Part model, mm, in its own coordinate system. A direction names the side the tool comes from. Give positions to 0.01 mm unless a question says otherwise; leave off trailing zeros. Order: outer loops, then holes, each group sorted by start corner. A loop starts at its lowest first (then second) coordinate and runs counter-clockwise, first axis right, second up. Notation, with made-up numbers: M -3.75,73.5 L 35.25,73.5 A20 ccw 35.25,90.5 Z; hole C 78,35.25 d10. An arc over 180 degrees is marked long. One line per question, with ' | ' between items.
```python
from build123d import *

# Parameters (mm, degrees)
F1_DEPTH  = 76.2
F2_DEPTH  = 12.7
F3_R      = 76.19999
F6_DEPTH  = 25.401
F7_DEPTH  = 25.401
F5_W      = 38.1
F5_H      = 12.7
F5_H_2    = 25.4
F8_DEPTH  = 25.4
F9_R      = 25.4
F10_R     = 25.39999
F11_DEPTH = 12.7


# Not quite as in the source:
# - a fillet or chamfer is up to 0.001 mm smaller than in the source, because OpenCascade refuses the exact size
# - a feature names something its author has since deleted; it is built from what else it names


with BuildPart() as f1:
    # F0 (on Front) → F1 (new body, symmetric)
    with BuildSketch(Plane.XZ):
        Polygon((0, 203.2), (0, 0), (254, 0), (254, 25.4), (76.2, 25.4), (25.4, 25.4), (25.4, 76.2), (25.4, 203.2), align=None)
    extrude(amount=F1_DEPTH, both=True)

    # F0 (on Front) → F2 (join, symmetric)
    with BuildSketch(Plane.XZ):
        Polygon((76.2, 25.4), (25.4, 76.2), (25.4, 25.4), align=None)
    extrude(amount=F2_DEPTH, both=True)

    # F3 (radius 76.2 in the source; OpenCascade refuses exactly that, so slightly less here)
    f3_edges = [f1.edges().sort_by_distance(p)[0] for p in [
        (12.7, -76.2, 203.2),
        (12.7, 76.2, 203.2),
    ]]
    fillet(f3_edges, radius=F3_R)

    # F5 (on face) → F6 (cut, through all)
    with BuildSketch(Plane.XY.offset(25.4)):
        with BuildLine():
            Line((203.2, 63.5), (127, 63.5))
            ThreePointArc((127, 63.5), (114.3, 50.8), (127, 38.1))
            Line((127, 38.1), (203.2, 38.1))
            ThreePointArc((203.2, 38.1), (215.9, 50.8), (203.2, 63.5))
        make_face()
        with BuildLine():
            Line((203.2, -38.1), (127, -38.1))
            ThreePointArc((127, -38.1), (114.3, -50.8), (127, -63.5))
            Line((127, -63.5), (203.2, -63.5))
            ThreePointArc((203.2, -63.5), (215.9, -50.8), (203.2, -38.1))
        make_face()
    extrude(amount=-F6_DEPTH, mode=Mode.SUBTRACT)

    # F4 (on face) → F7 (cut, through all)
    with BuildSketch(Plane.YZ.offset(25.4)):
        with BuildLine():
            Line((0, 101.6), (0, 177.8))
            ThreePointArc((0, 177.8), (-38.1, 139.7), (0, 101.6))
        make_face()
        with BuildLine():
            ThreePointArc((0, 101.6), (26.9407683632, 112.7592316368), (38.1, 139.7))
            ThreePointArc((38.1, 139.7), (26.9407683632, 166.6407683632), (0, 177.8))
            Line((0, 177.8), (0, 101.6))
        make_face()
    extrude(amount=-F7_DEPTH, mode=Mode.SUBTRACT)

    # F5 (on face) → F8 (join)
    with BuildSketch(Plane.XY.offset(25.4)):
        with Locations((273.05, 19.05)):
            Rectangle(F5_W, F5_H)
        with Locations((273.05, -19.05)):
            Rectangle(F5_W, F5_H)
        with Locations((273.05, 0)):
            Rectangle(F5_W, F5_H_2)
    extrude(amount=-F8_DEPTH)

    # F9
    f9_edges = [f1.edges().sort_by_distance(p)[0] for p in [
        (254, 76.2, 12.7),
        (254, -76.2, 12.7),
    ]]
    fillet(f9_edges, radius=F9_R)

    # F10 (radius 25.4 in the source; OpenCascade refuses exactly that, so slightly less here)
    f10_edges = [f1.edges().sort_by_distance(p)[0] for p in [
        (254, 25.4, 12.7),
        (254, -25.4, 12.7),
    ]]
    fillet(f10_edges, radius=F10_R)

    # F5 (on face) → F11 (cut)
    with BuildSketch(Plane.XY.offset(25.4)):
        with BuildLine():
            Line((254, -12.7), (254, 12.7))
            ThreePointArc((254, 12.7), (241.3, 0), (254, -12.7))
        make_face()
        with Locations((273.05, 0)):
            Rectangle(F5_W, F5_H_2)
    extrude(amount=-F11_DEPTH, mode=Mode.SUBTRACT)


solid = f1.part
```
1. Mould opens along Y. For faces 6 (the cylindrical face through (114.303, 51.079, 12.878)), 7 (the flat face through (51.2, -0.2, 50.4)), 8 (the cylindrical face through (246.36, 68.96, 12.88)) say: released by +Y, released by -Y, zero draft, split by the parting line, or undercut.
Worked out:
face 6: undercut | face 7: zero draft | face 8: released by +Y
2. Drop flat-ended pins along their axis: pin 1 (3 mm diameter, centred on x = 87, y = -22, fed in from +Z); pin 2 (14 mm diameter, centred on x = 286.5, z = 15.5, fed in from -Y); pin 3 (6.5 mm diameter, centred on x = 271, z = 20, fed in from +Y). Give the stop position or say it passes through.
Worked out:
pin 1: stops at z = 25.4 | pin 2: stops at y = -25.4 | pin 3: stops at y = 28.23
3. Tool access for faces 1 (the flat face through (39, 12.7, 40)), 2 (the flat face through (161, -1, 25.4)), 3 (the flat face through (71, 76.2, 21)), 4 (the flat face through (166, 63.5, 13)), 5 (the flat face through (286, -25.4, 13)): list every direction of +Z, -Z, +X, -X, +Y, -Y with a clear straight run to the whole face (end or side of a thin tool).
Worked out:
face 1: +Z, +X, +Y | face 2: +Z, +X | face 3: +Z, -Z, +X, -X, +Y | face 4: +Z, -Z | face 5: +Z, -Z, +X, -Y
4. Slice it at A-A on x = 184. Give the cut face in (y, z), then the cut area to 3 significant figures.
Worked out:
outline: M -76.2,0 L -63.5,0 L -63.5,25.4 L -76.2,25.4 Z; M -38.1,0 L 38.1,0 L 38.1,25.4 L -38.1,25.4 Z; M 63.5,0 L 76.2,0 L 76.2,25.4 L 63.5,25.4 Z | area: 2,580 mm2
5. Slice it at B-B on z = 144. Give the cut face in (x, y).
Worked out:
outline: M 0,-74.28 L 25.4,-74.28 L 25.4,-37.86 L 0,-37.86 Z; M 0,37.86 L 25.4,37.86 L 25.4,74.28 L 0,74.28 Z
6. Slice it at D-D on x = 59.5. Give the cut face in (y, z), then the cut area to 3 significant figures.
Worked out:
outline: M -76.2,0 L 76.2,0 L 76.2,25.4 L 12.7,25.4 L 12.7,42.1 L -12.7,42.1 L -12.7,25.4 L -76.2,25.4 Z | area: 4,300 mm2
7. Slice it at C-C on y = -17. Give the cut face in (x, z), then the cut area to 3 significant figures.
Worked out:
outline: M 0,0 L 292.1,0 L 292.1,25.4 L 25.4,25.4 L 25.4,105.6 L 0,105.6 Z; M 0,173.8 L 25.4,173.8 L 25.4,201.28 L 0,201.28 Z | area: 10,200 mm2
8. Probe L1, parallel to X at y = 48, z = 127.5; L2, parallel to Y at x = 249, z = 19.5; L3, parallel to Y at x = 10.75, z = 139.7. List the from-to ranges inside material, lowest first. Write a range as from..to.
Worked out:
L1: x = 0..25.4 | L2: y = -65.93..-11.67, 11.67..65.93 | L3: y = -75.13..-38.1, 38.1..75.13
